from build123d import *

# Parameters (mm, degrees)
SKETCH1_W                 = 50.705
SKETCH1_H                 = 42.455
SKETCH1_R                 = 1.65288
BOSS_EXTRUDE1_DEPTH       = 3.5
SKETCH2_W                 = 46.705
SKETCH2_H                 = 38.455
CUT_EXTRUDE1_DEPTH        = 2.024
SKETCH3_R                 = 6
SKETCH3_R_2               = 3.625
BOSS_EXTRUDE2_DEPTH       = 3.5
FILLET2_R                 = 1.5
FILLET3_R                 = 1
MIRROR2_COPY_1_SKETCH_R   = 6
MIRROR2_COPY_1_SKETCH_R_2 = 3.625
MIRROR2_COPY_1_DEPTH      = 3.5
FILLET1_R                 = 10


with BuildPart() as part:
    # Sketch1 → Boss-Extrude1 (new body)
    with BuildSketch(Plane(origin=(0, 0, 0), x_dir=(1, 0, 0), z_dir=(0, 1, 0))):
        Rectangle(SKETCH1_W, SKETCH1_H)
        with Locations(Location((-19.995, 15.87, 0), (0, 0, 270))):
            Circle(SKETCH1_R, mode=Mode.SUBTRACT)
        with Locations(Location((19.995, 15.87, 0), (0, 0, 90))):
            Circle(SKETCH1_R, mode=Mode.SUBTRACT)
        with Locations(Location((19.995, -15.87, 0), (0, 0, 270))):
            Circle(SKETCH1_R, mode=Mode.SUBTRACT)
        with Locations(Location((-19.995, -15.87, 0), (0, 0, 90))):
            Circle(SKETCH1_R, mode=Mode.SUBTRACT)
        with BuildLine():
            Line((21.8525, 13.0125), (21.8525, -13.0125))
            Line((21.8525, -13.0125), (19.995, -13.0125))
            ThreePointArc((19.995, -13.0125), (17.974442373, -13.849442373), (17.1375, -15.87))
            Line((17.1375, -15.87), (17.1375, -17.7275))
            Line((17.1375, -17.7275), (-17.1375, -17.7275))
            Line((-17.1375, -17.7275), (-17.1375, -15.87))
            ThreePointArc((-17.1375, -15.87), (-17.974442373, -13.849442373), (-19.995, -13.0125))
            Line((-19.995, -13.0125), (-21.8525, -13.0125))
            Line((-21.8525, -13.0125), (-21.8525, 13.0125))
            Line((-21.8525, 13.0125), (-19.995, 13.0125))
            ThreePointArc((-19.995, 13.0125), (-17.974442373, 13.849442373), (-17.1375, 15.87))
            Line((-17.1375, 15.87), (-17.1375, 17.7275))
            Line((-17.1375, 17.7275), (17.1375, 17.7275))
            Line((17.1375, 17.7275), (17.1375, 15.87))
            ThreePointArc((17.1375, 15.87), (17.974442373, 13.849442373), (19.995, 13.0125))
            Line((19.995, 13.0125), (21.8525, 13.0125))
        make_face(mode=Mode.SUBTRACT)
    extrude(amount=BOSS_EXTRUDE1_DEPTH)

    # Sketch2 → Cut-Extrude1 (cut)
    with BuildSketch(Plane(origin=(0, 3.5, 0), x_dir=(1, 0, 0), z_dir=(0, 1, 0))):
        Rectangle(SKETCH2_W, SKETCH2_H)
    extrude(amount=-CUT_EXTRUDE1_DEPTH, mode=Mode.SUBTRACT)

    # Sketch3 → Boss-Extrude2 (add)
    # profile 1 of 3: a face of its own
    with BuildSketch(Plane(origin=(0, 3.5, 0), x_dir=(1, 0, 0), z_dir=(0, 1, 0))):
        with BuildLine():
            Line((-25.3525, 21.2275), (-21.403966459, 21.2275))
            Line((-21.403966459, 21.2275), (-34.48647943, 35.98289392))
            ThreePointArc((-34.48647943, 35.98289392), (-35.995113658, 33.91607267), (-38.227727219, 32.665807098))
            Line((-38.227727219, 32.665807098), (-25.3525, 18.144204877))
            Line((-25.3525, 18.144204877), (-25.3525, 21.2275))
        make_face()
    # profile 2 of 3: a face of its own
    with BuildSketch(Plane(origin=(0, 3.5, 0), x_dir=(1, 0, 0), z_dir=(0, 1, 0))):
        Polygon((-23.891843474, 20.265138811), (-20.550712197, 20.265138811), (-21.403966459, 21.2275), (-25.3525, 21.2275), (-25.3525, 18.144204877), (-24.536212364, 17.223537292), align=None)
    # profile 3 of 3: a face of its own
    with BuildSketch(Plane(origin=(0, 3.5, 0), x_dir=(1, 0, 0), z_dir=(0, 1, 0))):
        with Locations((-39.975617845, 38.405570016)):
            Circle(SKETCH3_R)
        with Locations(Location((-39.975617845, 38.405570016, 0), (0, 0, 270))):
            Circle(SKETCH3_R_2, mode=Mode.SUBTRACT)
    boss_extrude2 = extrude(amount=-BOSS_EXTRUDE2_DEPTH)

    # Fillet2
    fillet2_edges = [part.edges().sort_by_distance(p)[0] for p in [
        (21.8525, 0.738, -13.0125),
        (21.8525, 0.738, 13.0125),
        (17.1375, 0.738, 17.7275),
        (-17.1375, 0.738, 17.7275),
        (-21.8525, 0.738, 13.0125),
        (-21.8525, 0.738, -13.0125),
        (-17.1375, 0.738, -17.7275),
        (17.1375, 0.738, -17.7275),
    ]]
    fillet(fillet2_edges, radius=FILLET2_R)

    # Fillet3
    fillet3_edges = [part.edges().sort_by_distance(p)[0] for p in [
        (-23.3525, 2.488, 19.2275),
        (-23.3525, 2.488, -19.2275),
        (23.3525, 2.488, -19.2275),
        (23.3525, 2.488, 19.2275),
    ]]
    fillet(fillet3_edges, radius=FILLET3_R)

    # Mirror1: Boss-Extrude2 across plane
    add(boss_extrude2.mirror(Plane.XY))

    # Mirror2: Boss-Extrude2 across plane
    add(boss_extrude2.mirror(Plane(origin=(0, 0, 0), x_dir=(0, 0, 1), z_dir=(1, 0, 0))))

    # Mirror2 copy 1 sketch → Mirror2 copy 1 (add)
    # profile 1 of 3: a face of its own
    with BuildSketch(Plane(origin=(0, 3.5, 0), x_dir=(-1, 0, 0), z_dir=(0, 1, 0))):
        with BuildLine():
            Line((-25.3525, 21.2275), (-21.403966459, 21.2275))
            Line((-21.403966459, 21.2275), (-34.48647943, 35.98289392))
            ThreePointArc((-34.48647943, 35.98289392), (-35.995113658, 33.91607267), (-38.227727219, 32.665807098))
            Line((-38.227727219, 32.665807098), (-25.3525, 18.144204877))
            Line((-25.3525, 18.144204877), (-25.3525, 21.2275))
        make_face()
    # profile 2 of 3: a face of its own
    with BuildSketch(Plane(origin=(0, 3.5, 0), x_dir=(-1, 0, 0), z_dir=(0, 1, 0))):
        Polygon((-23.891843474, 20.265138811), (-20.550712197, 20.265138811), (-21.403966459, 21.2275), (-25.3525, 21.2275), (-25.3525, 18.144204877), (-24.536212364, 17.223537292), align=None)
    # profile 3 of 3: a face of its own
    with BuildSketch(Plane(origin=(0, 3.5, 0), x_dir=(-1, 0, 0), z_dir=(0, 1, 0))):
        with Locations((-39.975617845, 38.405570016)):
            Circle(MIRROR2_COPY_1_SKETCH_R)
        with Locations(Location((-39.975617845, 38.405570016, 0), (0, 0, 270))):
            Circle(MIRROR2_COPY_1_SKETCH_R_2, mode=Mode.SUBTRACT)
    extrude(amount=-MIRROR2_COPY_1_DEPTH)

    # Fillet1
    fillet1_edges = [part.edges().sort_by_distance(p)[0] for p in [
        (-25.3525, 1.75, -18.144204877),
        (-21.403966459, 1.75, -21.2275),
        (-34.48647943, 1.75, -35.98289392),
        (-38.227727219, 1.75, -32.665807098),
        (-21.403966459, 1.75, 21.2275),
        (-38.227727219, 1.75, 32.665807098),
        (-34.48647943, 1.75, 35.98289392),
        (-25.3525, 1.75, 18.144204877),
        (25.3525, 1.75, 18.144204877),
        (34.48647943, 1.75, 35.98289392),
        (38.227727219, 1.75, 32.665807098),
        (21.403966459, 1.75, 21.2275),
        (21.403966459, 1.75, -21.2275),
        (38.227727219, 1.75, -32.665807098),
        (34.48647943, 1.75, -35.98289392),
        (25.3525, 1.75, -18.144204877),
    ]]
    fillet(fillet1_edges, radius=FILLET1_R)


solid = part.part
Read the model definition and answer for the solid it produces. Units are mm, in the model's axes. A direction names the side the tool comes from. Give positions to 0.01 mm unless a question says otherwise; leave off trailing zeros. Write each loop counter-clockwise with the first axis right and the second up, starting at its lowest first coordinate (ties: lowest second). Pieces come first, ordered by that corner, then holes. Notation, with made-up numbers: (56.5, -21) - (76.5, -21) arc R10 ccw to (76.5, -8) - close; hole circle Ø1 at (88, 40.25). An arc over 180 degrees is marked (long way). Answer in a Markdown table with one row per item. Add a question column.
Item 1: Find the intervals of material crossed by L1, parallel to Z at x = 3, y = 2.8; L2, parallel to X at y = 0.5, z = 11.5; L3, parallel to X at y = 2.6, z = 11, in increasing order.
Item 2: Section C-C, the plane x = 26.5 is taken. Write down the section's boundary in (y, z).
Item 3: Section B-B, the plane z = 31 is taken. Write down the section's boundary in (x, y).
Item 4: Determine the mould class of faces 6 (the face through (33.234, 1.726, 35.395)), 7 (the face through (-36.919, 1.774, 36.457)), 8 (the face through (37.79, 1.73, 31.35)), 9 (the face through (27.884, 1.774, -28.536)) for opening direction Z: pulls with the +Z half, pulls with the -Z half, needs draft (parallel to the pull), parting line crosses it, or undercut.
Item 5: Flat-ended cylindrical pins translate along their axes: P1, Ø0.7, axis at y = 1, z = -1, coming from the +X side; P2, Ø1, axis at x = -4.5, y = 3, coming from the -Z side; P3, Ø1.6, axis at x = -0.5, y = 1, coming from the +Z side; P4, Ø2, axis at x = -19.995, z = -15.87, coming from the +Y side. Find the tip coordinate at first contact, or state that the pin passes through.
Item 6: Section A-A, the plane x = -0.5 is taken. Write down the section's boundary in (y, z).
Item 7: A tool of negligible diameter and unlimited length cuts with its end or side. For faces 1 (the face through (-21.06, 1.73, 22.13)), 2 (the face through (26.02, 1.73, -17.94)), 3 (the face through (17.997, 0.728, 13.827)), 4 (the face through (-25.352, 2, 0)), 5 (the face through (33.234, 1.726, -35.395)), from which of +Z, -Z, +X, -X, +Y, -Y can it reach the whole face along a straight path? Write none if from no direction.
Recorded:
| question | item | result |
|---|---|---|
| 1 | L1 | z = -21.23 to -19.23, 19.23 to 21.23 |
| 1 | L2 | x = -25.35 to -21.85, 21.85 to 25.35 |
| 1 | L3 | x = -25.35 to -23.35, 23.35 to 25.35 |
| 2 | outline | (0, -26.98) - (3.5, -26.98) - (3.5, -19) - (0, -19) - close; (0, 19) - (3.5, 19) - (3.5, 26.98) - (0, 26.98) - close |
| 3 | outline | (-37.22, 0) - (-30.07, 0) - (-30.07, 3.5) - (-37.22, 3.5) - close; (30.07, 0) - (37.22, 0) - (37.22, 3.5) - (30.07, 3.5) - close |
| 4 | face 6 | pulls with the +Z half |
| 4 | face 7 | undercut |
| 4 | face 8 | undercut |
| 4 | face 9 | pulls with the -Z half |
| 5 | P1 | stops at x = 25.35 |
| 5 | P2 | stops at z = -21.23 |
| 5 | P3 | stops at z = 21.23 |
| 5 | P4 | passes through |
| 6 | outline | (0, -21.23) - (3.5, -21.23) - (3.5, -19.23) - (1.48, -19.23) - (1.48, -17.73) - (0, -17.73) - close; (0, 17.73) - (1.48, 17.73) - (1.48, 19.23) - (3.5, 19.23) - (3.5, 21.23) - (0, 21.23) - close |
| 7 | face 1 | +Z, +Y, -Y |
| 7 | face 2 | +X, +Y, -Y |
| 7 | face 3 | +Y, -Y |
| 7 | face 4 | -X, +Y, -Y |
| 7 | face 5 | -Z, +Y, -Y |
